Input: part model. Units: mm. Frame: model coordinates. Round coordinates to 2 decimals unless told otherwise and drop trailing zeros. Loops run counter-clockwise (first coordinate to the right, second up) from the corner with the lowest first, then second, coordinate; pieces in that order, holes last.
(1) Cut plane C-C, the plane x = 207.5. Output: boundary loops of the cut face in (y, z), and give its area (3 significant figures).
(2) First-contact query: pin 1 Ø8 at (x, y) = (-12, 16.5) entering from +Z; pin 2 Ø1.5 at (x, y) = (252.5, 29.5) entering from -Z. Flat tips, straight axial feed; report the tip coordinate or a pass-through.
(3) Cut plane A-A, the plane z = 766.5. Output: boundary loops of the cut face in (x, y), and give its area (3 significant figures).
(4) Cut plane B-B, the plane y = 27. Output: boundary loops of the cut face in (x, z), and give its area (3 significant figures).
(5) Line query: line 1 (Z direction, x = 189, y = 19.5); line 2 (X direction, y = -21, z = 115). Output: solid intervals per line, ascending.
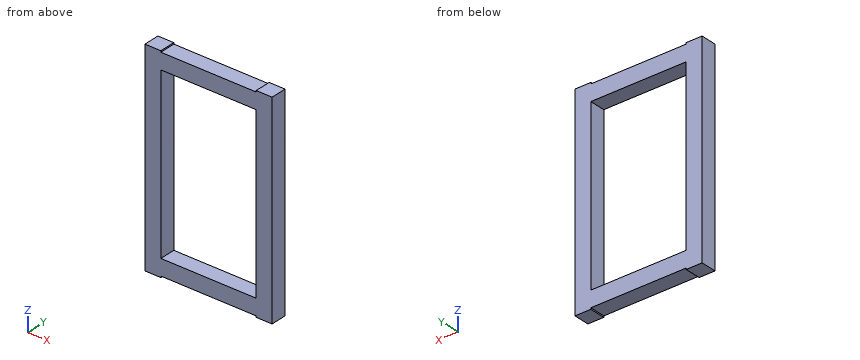
from build123d import *

# Parameters (mm, degrees)
F0_W      = 457.2
F0_H      = 76.2
F1_DEPTH  = 76.2
F1_FACE_W = 76.2
F1_FACE_H = 76.2
F2_DEPTH  = 152.4
F3_W      = 76.2
F3_H      = 76.2
F4_DEPTH  = 895.35
F5_W      = 76.2
F5_H      = 76.2
F11_DEPTH = 6.35
F6_W      = 76.2
F6_H      = 76.2
F7_DEPTH  = 533.4
F8_W      = 76.2
F8_H      = 76.2
F12_DEPTH = 895.35
F9_W      = 76.2
F9_H      = 76.2
F10_DEPTH = 6.35


with BuildPart() as f1:
    # F0 (on Top) → F1 (new body)
    with BuildSketch(Plane.XY):
        with Locations((4.465946, 3.0175)):
            Rectangle(F0_W, F0_H)
    extrude(amount=F1_DEPTH)

    # F1_face (on face) → F2 (join)
    with BuildSketch(Plane(origin=(233.065946, 3.0175, 38.1), x_dir=(0, 1, 0), z_dir=(1, 0, 0))):
        Rectangle(F1_FACE_W, F1_FACE_H)
    extrude(amount=F2_DEPTH)

    # F3 (on face) → F4 (join)
    with BuildSketch(Plane.XY.offset(76.2)):
        with Locations((347.365946, 3.0175)):
            Rectangle(F3_W, F3_H)
    extrude(amount=F4_DEPTH)

    # F5 (on face) → F11 (join)
    with BuildSketch(Plane(origin=(0, 0, 0), x_dir=(1, 0, 0), z_dir=(0, 0, -1))):
        with Locations((347.365946, -3.0175)):
            Rectangle(F5_W, F5_H)
    extrude(amount=F11_DEPTH)

    # F6 (on face) → F7 (join)
    with BuildSketch(Plane(origin=(309.265946, 0, 0), x_dir=(0, -1, 0), z_dir=(-1, 0, 0))):
        with Locations((-3.0175, 927.1)):
            Rectangle(F6_W, F6_H)
    extrude(amount=F7_DEPTH)

    # F8 (on face) → F12 (join)
    with BuildSketch(Plane(origin=(0, 0, 889), x_dir=(1, 0, 0), z_dir=(0, 0, -1))):
        with Locations((-186.034054, -3.0175)):
            Rectangle(F8_W, F8_H)
    extrude(amount=F12_DEPTH)

    # F9 (on face) → F10 (join)
    with BuildSketch(Plane.XY.offset(965.2)):
        with Locations((-186.034054, 3.0175)):
            Rectangle(F9_W, F9_H)
    extrude(amount=F10_DEPTH)


solid = f1.part
Reported:
1. outline: (-35.08, 0) - (41.12, 0) - (41.12, 76.2) - (-35.08, 76.2) - close; (-35.08, 889) - (41.12, 889) - (41.12, 965.2) - (-35.08, 965.2) - close
1. area: 11,600 mm2
2. pin 1: stops at z = 965.2
2. pin 2: stops at z = 0
3. outline: (-224.13, -35.08) - (-147.93, -35.08) - (-147.93, 41.12) - (-224.13, 41.12) - close; (309.27, -35.08) - (385.47, -35.08) - (385.47, 41.12) - (309.27, 41.12) - close
3. area: 11,600 mm2
4. outline: (-224.13, -6.35) - (-147.93, -6.35) - (-147.93, 0) - (309.27, 0) - (309.27, -6.35) - (385.47, -6.35) - (385.47, 971.55) - (309.27, 971.55) - (309.27, 965.2) - (-147.93, 965.2) - (-147.93, 971.55) - (-224.13, 971.55) - close; hole (-147.93, 76.2) - (309.27, 76.2) - (309.27, 889) - (-147.93, 889) - close
4. area: 219,000 mm2
5. line 1: z = 0 to 76.2, 889 to 965.2
5. line 2: x = -224.13 to -147.93, 309.27 to 385.47
